Autodesk Inventor part; units mm, degrees
ref_plane "YZ Plane" through (0, 0, 0) normal (1, 0, 0) x (0, 1, 0)
ref_plane "XZ Plane" through (0, 0, 0) normal (0, 1, 0) x (-1, 0, 0)
ref_plane "XY Plane" through (0, 0, 0) normal (0, 0, 1) x (1, 0, 0)
sketch "Sketch1" plane through (0, 0, 0) normal (0, 1, 0) x (-1, 0, 0)
  line L0 (9.02, 19.685) -> (-9.02, 19.685)
  line L1 (-9.02, 19.685) -> (-9.02, -19.685)
  line L2 (-9.02, -19.685) -> (9.02, -19.685)
  line L3 (9.02, -19.685) -> (9.02, 19.685)
  circle A0 centre (4.51, 16.6309) radius 1.4224
  circle A1 centre (-4.51, 16.6309) radius 1.4224
  circle A2 centre (4.51, -16.6309) radius 1.4224
  circle A3 centre (-4.51, -16.6309) radius 1.4224
  point P0 (0, 0)
  dimension "d0" = 39.37
  dimension "d1" = 19.685
  dimension "d2" = 18.04
  dimension "d3" = 9.02
  dimension "d4" = 4.51
  dimension "d5" = 3.0541
  dimension "d6" = 2.8448
  dimension "d7" = 3.0541
  dimension "d8" = 3.0541
  dimension "d9" = 3.0541
  dimension "d10" = 2.8448
  dimension "d11" = 2.8448
  dimension "d12" = 2.8448
  dimension "d13" = 4.51
  dimension "d14" = 4.51
  dimension "d15" = 4.51
extrude "Extrusion1" add sketch "Sketch1" along normal blind 6.35
equation "\"d7\" = d5"
equation "\"d8\" = d5"
equation "\"d9\" = d5"
equation "\"d10\" = d6"
equation "\"d11\" = d10"
equation "\"d12\" = d6"
equation "\"d13\" = d4"
equation "\"d14\" = d4"
equation "\"d15\" = d4"
properties part number "MotorMountSpacer" material "Aluminum 6061"
Work out the finished part from the listing and answer in its coordinate system (mm). Coordinates: 2 decimals unless noted, no trailing zeros. Write each loop counter-clockwise with the first axis right and the second up, starting at its lowest first coordinate (ties: lowest second). Pieces come first, ordered by that corner, then holes. Notation, with made-up numbers: (62.25, -34.75) - (98.25, -34.75) arc R22 cw to (98.25, -28.75) - close; hole circle Ø11 at (-27.75, 73.25). An arc over 180 degrees is marked (long way). Answer as a JSON object with one key per item and string values.
Q1. Find section B-B (y = 4.5). Write down the section's boundary in (x, z) (3 decimals), plus the area to 3 significant figures.
Results list:
{"outline": "(-9.02, -19.685) - (9.02, -19.685) - (9.02, 19.685) - (-9.02, 19.685) - close; hole circle Ø2.845 at (-4.51, -16.631); hole circle Ø2.845 at (-4.51, 16.631); hole circle Ø2.845 at (4.51, -16.631); hole circle Ø2.845 at (4.51, 16.631)", "area": "685 mm^2"}
Q2. Consider L1, parallel to Z at x = -4.51, y = 3.5 (1 decimal); L2, parallel to Z at x = 3.25, y = 4.25 (3 decimals). Determine where each line is inside the solid, lowest interval first. Write a range as from..to.
Results list:
{"L1": "z = -19.7..-18.1, -15.2..15.2, 18.1..19.7", "L2": "z = -19.685..-17.291, -15.971..15.971, 17.291..19.685"}
Q3. For a pull along X with two mould halves and no side action, classify faces 1 (the flat face through (0, 6.35, 0)), 2 (the flat face through (-9.02, 3, 0)), 3 (the flat face through (9.02, 3, 0)), 4 (the cylindrical face through (3.7, 3.1, -17.8)) as pulls with the +X half, pulls with the -X half, needs draft (parallel to the pull), parting line crosses it, or undercut.
Results list:
{"face 1": "needs draft", "face 2": "pulls with the -X half", "face 3": "pulls with the +X half", "face 4": "undercut"}
Q4. Find section A-A (x = 4.51). State how many separate pieces and enclosed holes the cut face has, plus the area to 3 significant figures.
Results list:
{"separate pieces": "3", "enclosed holes": "0", "area": "214 mm^2"}
